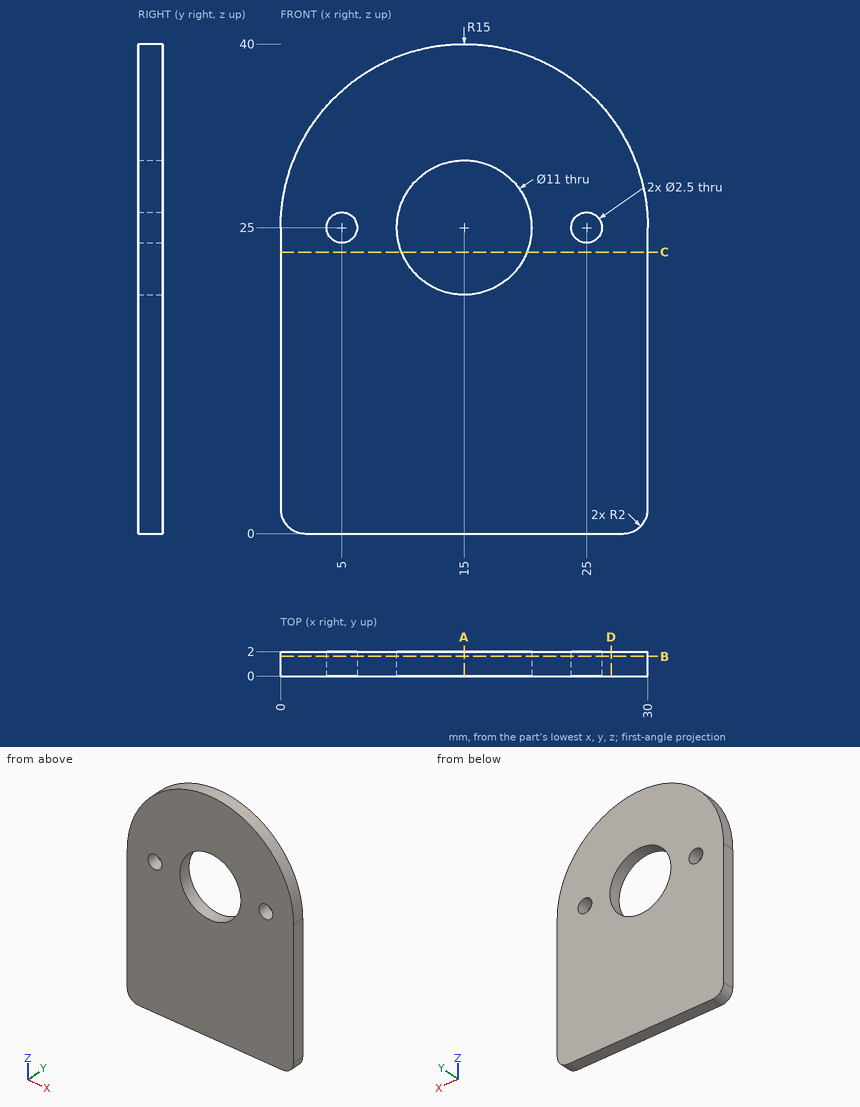
Here's the drawing with two shaded views (mm, measured from the low corner). I have some questions. Give positions to 0.01 mm unless a question says otherwise; leave off trailing zeros. Write each loop counter-clockwise with the first axis right and the second up, starting at its lowest first coordinate (ties: lowest second). Pieces come first, ordered by that corner, then holes. Notation, with made-up numbers: (-10, 54) -> (2, 54) arc R18 cw to (2, 69) -> close; hole circle Ø2 at (-36, 15.5). An arc over 180 degrees is marked (long way). Use one line per item in the form item = value. Start each with the question number.
1. Imagine slicing it at B-B on y = 1.6. List the corners of the cut face in (x, z) for me, plus the area to 3 significant figures.
2. Imagine slicing it at D-D on x = 27. List the corners of the cut face in (y, z) for me.
3. Imagine slicing it at C-C on z = 23. List the corners of the cut face in (x, y) for me.
4. Imagine slicing it at A-A on x = 15. List the corners of the cut face in (y, z) for me.
5. Will this pin go through, and if not, where does the flat tip stop? pin 1 Ø2 at (x, z) = (25, 25) entering from -Y.
6. If I drill on L1, parallel to X at y = 1.55, z = 25; L2, parallel to Z at x = 15, y = 1; L3, parallel to Z at x = 5, y = 0.45, over which ranges is the centre line in solid material (lowest first)?
Entries:
q1.outline = (0, 2) arc R2 ccw to (2, 0) -> (28, 0) arc R2 ccw to (30, 2) -> (30, 25) arc R15 ccw to (0, 25) -> close; hole circle Ø2.5 at (5, 25); hole circle Ø11 at (15, 25); hole circle Ø2.5 at (25, 25)
q1.area = 997 mm²
q2.outline = (0, 0) -> (2, 0) -> (2, 34) -> (0, 34) -> close
q3.outline = (0, 0) -> (9.88, 0) -> (9.88, 2) -> (0, 2) -> close; (20.12, 0) -> (30, 0) -> (30, 2) -> (20.12, 2) -> close
q4.outline = (0, 0) -> (2, 0) -> (2, 19.5) -> (0, 19.5) -> close; (0, 30.5) -> (2, 30.5) -> (2, 40) -> (0, 40) -> close
q5.pin_1 = through
q6.L1 = 0 to 3.75, 6.25 to 9.5, 20.5 to 23.75, 26.25 to 30
q6.L2 = 0 to 19.5, 30.5 to 40
q6.L3 = 0 to 23.75, 26.25 to 36.18
